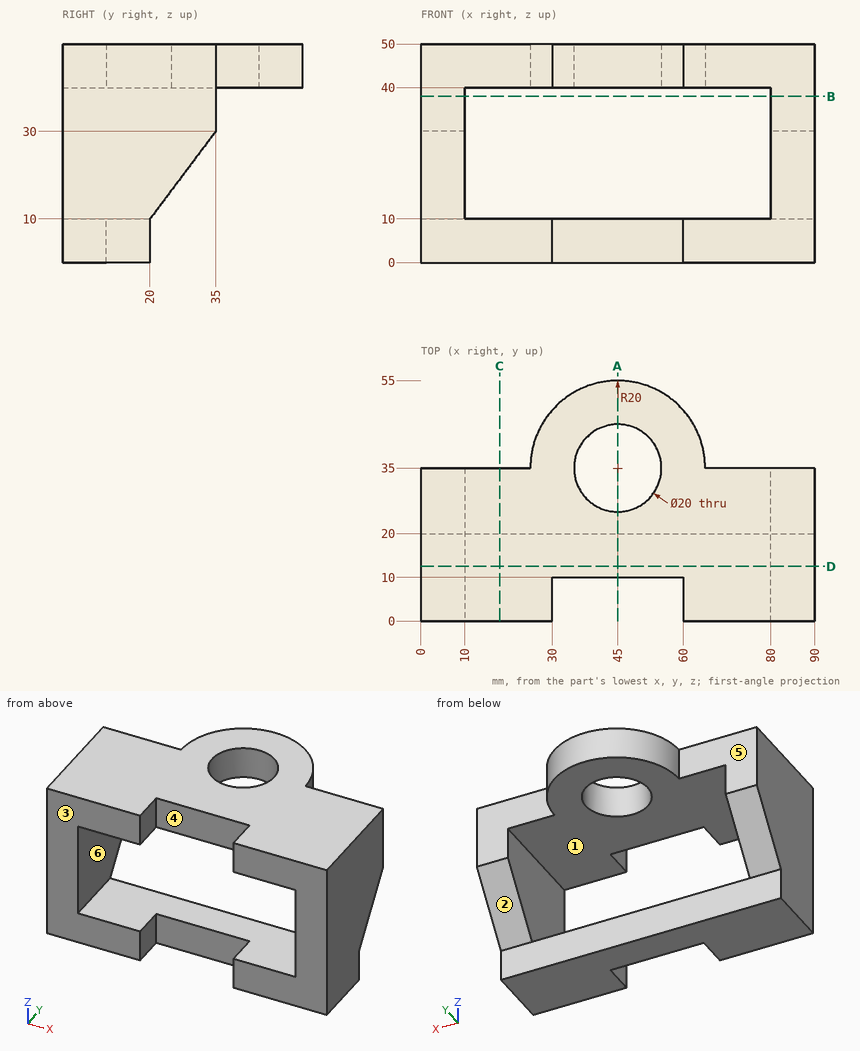
Check sheet for the drawn part. Datum: minimum x, y, z corner. Units: mm. A direction names the side the tool comes from. Give positions to 0.01 mm unless a question says otherwise; leave off trailing zeros. Write each loop counter-clockwise with the first axis right and the second up, starting at its lowest first coordinate (ties: lowest second). Pieces come first, ordered by that corner, then holes.
(1) Mould release check, pull along Z, two halves, no side actions. Record for the marked faces 1, 2 and 3: +Z half, -Z half, draft (parallel to the pull), parting line (faces both ways), or undercut.
(2) Cross-section at D-D (y = 12.5). Enter the section's corners in (x, z).
(3) Gauge pin test, flat ends, axial feed: pin 1 (6 mm diameter, centred on x = 11, z = 41, fed in from +Y); pin 2 (1 mm diameter, centred on x = 63.5, y = 39.5, fed in from -Z); pin 3 (5 mm diameter, centred on x = 48.5, z = 44.5, fed in from -Y). Record the tip position at first contact, or that the pin passes through.
(4) Cross-section at B-B (z = 38). Enter the section's corners in (x, y), plus the area to 3 significant figures.
(5) Cross-section at A-A (x = 45). Enter the section's corners in (y, z).
(6) Cross-section at C-C (x = 18). Enter the section's corners in (y, z).
(7) Material ranges on line 1 (Y direction, x = 45, z = 42.75); line 2 (Z direction, x = 49.5, y = 14); line 3 (X direction, y = 34.5, z = 33), recorded low to high.
(8) Access from +Z, -Z, +X, -X, +Y, -Y to the whole of each face (thin tool, end or side, straight path). Record for the marked faces 4, 5 and 6.
Worked out:
1. face 1: undercut
1. face 2: -Z half
1. face 3: draft
2. outline: (0, 0) - (90, 0) - (90, 50) - (0, 50) - close; hole (10, 10) - (80, 10) - (80, 40) - (10, 40) - close
3. pin 1: stops at y = 35
3. pin 2: stops at z = 40
3. pin 3: stops at y = 10
4. outline: (0, 0) - (10, 0) - (10, 35) - (0, 35) - close; (80, 0) - (90, 0) - (90, 35) - (80, 35) - close
4. area: 700 mm2
5. outline: (10, 0) - (20, 0) - (20, 10) - (10, 10) - close; (10, 40) - (25, 40) - (25, 50) - (10, 50) - close; (45, 40) - (55, 40) - (55, 50) - (45, 50) - close
6. outline: (0, 0) - (20, 0) - (20, 10) - (0, 10) - close; (0, 40) - (35, 40) - (35, 50) - (0, 50) - close
7. line 1: y = 10 to 25, 45 to 55
7. line 2: z = 0 to 10, 40 to 50
7. line 3: x = 0 to 10, 80 to 90
8. face 4: +Z, -Z, -Y
8. face 5: +Z, -Z, -X, +Y
8. face 6: +Y, -Y
